from build123d import *

# Parameters (mm, degrees)
F1_DEPTH = 3.556


with BuildPart() as f1:
    # F0 (on Top) → F1 (new body)
    with BuildSketch(Plane.XY):
        Polygon((0, 374.65), (0, 0), (539.75, 0), (539.75, 374.65), (416.483468, 374.65), (123.825, 374.65), align=None)
        with BuildLine():
            ThreePointArc((120.653815, 330.36432), (121.635642, 332.508135), (123.825, 333.383715))
            ThreePointArc((123.825, 333.383715), (126.070064, 332.453779), (127, 330.208715))
            Line((127, 330.208715), (127, 313.663327))
            ThreePointArc((127, 313.663327), (123.822934, 297.788327), (120.653815, 313.664915))
            Line((120.653815, 313.664915), (120.653815, 330.05311))
            ThreePointArc((120.653815, 330.05311), (120.65, 330.208715), (120.653815, 330.36432))
        make_face(mode=Mode.SUBTRACT)
        with BuildLine():
            ThreePointArc((413.311554, 330.348675), (414.288445, 332.502729), (416.483468, 333.383715))
            ThreePointArc((416.483468, 333.383715), (418.708128, 332.473999), (419.657948, 330.266165))
            ThreePointArc((419.657948, 330.266165), (419.658468, 330.208715), (419.657948, 330.151265))
            Line((419.657948, 330.151265), (419.657948, 313.663543))
            ThreePointArc((419.657948, 313.663543), (416.482078, 297.788327), (413.311554, 313.664612))
            Line((413.311554, 313.664612), (413.311554, 330.068754))
            ThreePointArc((413.311554, 330.068754), (413.308468, 330.208715), (413.311554, 330.348675))
        make_face(mode=Mode.SUBTRACT)
    extrude(amount=F1_DEPTH)


solid = f1.part
Can you work these out from the model? Positions are in its coordinate system, mm. Coordinates: 2 decimals unless noted, no trailing zeros. Order: outer loops, then holes, each group sorted by start corner. A loop starts at its lowest first (then second) coordinate and runs counter-clockwise, first axis right, second up. Notation, with made-up numbers: M 49,89 L 86,89 A25 cw 86,102 Z; hole C 83,-11.75 d4. An arc over 180 degrees is marked long. Write item = value, one per line.
(1) If we mould it in two halves opening along Y, with no side actions, what happens to faces 1 (the face through (124.14, 297.794, 1.753)), 2 (the face through (416.799, 297.794, 1.753)), 3 (the face through (266, 190, 3.556))? For each: pulls with the +Y half, pulls with the -Y half, needs draft (parallel to the pull), parting line crosses it, or undercut.
Results are:
face_1 = undercut
face_2 = undercut
face_3 = needs draft
(2) Suppose I cut it at A-A on y = 305.5. Please give me the cut outline in (x, z).
Results are:
outline = M 0,0 L 115.59,0 L 115.59,3.56 L 0,3.56 Z; M 132.06,0 L 408.25,0 L 408.25,3.56 L 132.06,3.56 Z; M 424.72,0 L 539.75,0 L 539.75,3.56 L 424.72,3.56 Z
(3) For pin 1 Ø15 at (x, y) = (123.83, 306.04) entering from -Z, with a flat end and sliding along its axis, tell me the tip position at first contact or that it passes through.
Results are:
pin_1 = through
(4) I need wall thicknesses on line 1 along X through (y, z) = (324, 1.3); line 2 along X through (y, z) = (309.5, 1.4). Which ranges of each line are inside material? Lowest first, please. Write a range as [from, to].
Results are:
line_1 = [0, 120.65], [127, 413.31], [419.66, 539.75]
line_2 = [0, 116.33], [131.32, 408.99], [423.98, 539.75]
